Design review of the part built by this model. Coordinates are the model's own, in mm. A direction names the side the tool comes from. Coordinates: 2 decimals unless noted, no trailing zeros. Loops run counter-clockwise (first coordinate to the right, second up) from the corner with the lowest first, then second, coordinate; pieces in that order, holes last. Notation, with made-up numbers: (69, 37) -> (89, 37) arc R14 ccw to (89, 63) -> close; hole circle Ø11 at (-4, 6). An arc over 180 degrees is marked (long way). Use CSV: the item, a comma, the result in double quotes.
```python
from build123d import *

# Parameters (mm, degrees)
BOSS_EXTRUDE1_DEPTH = 10
SKETCH2_R           = 1.85
CUT_EXTRUDE1_DEPTH  = 40
SKETCH2_3_R         = 1.85
CUT_EXTRUDE2_DEPTH  = 40
BOSS_EXTRUDE2_DEPTH = 3


with BuildPart() as part:
    # Sketch1 → Boss-Extrude1 (new body)
    with BuildSketch(Plane.XY):
        Polygon((0, 26), (34.5, 26), (34.5, 0), (45.5, 0), (45.5, 7.020180644), (37.5, 29), (0, 29), align=None)
    extrude(amount=BOSS_EXTRUDE1_DEPTH)

    # Sketch2 → Cut-Extrude1 (cut)
    # profile 1 of 2: a face of its own
    with BuildSketch(Plane(origin=(0, 7.020180644, 0), x_dir=(1, 0, 0), z_dir=(0, 1, 0))):
        Polygon((37, -3.267949192), (37, -6.732050808), (40, -8.464101615), (43, -6.732050808), (43, -3.267949192), (40, -1.535898385), align=None)
        with Locations((40, -5)):
            Circle(SKETCH2_R, mode=Mode.SUBTRACT)
    # profile 2 of 2: a face of its own
    with BuildSketch(Plane(origin=(0, 7.020180644, 0), x_dir=(1, 0, 0), z_dir=(0, 1, 0))):
        with Locations((40, -5)):
            Circle(SKETCH2_R)
    extrude(amount=CUT_EXTRUDE1_DEPTH, mode=Mode.SUBTRACT)

    # Sketch2_3 → Cut-Extrude2 (cut)
    with BuildSketch(Plane(origin=(0, 7.020180644, 0), x_dir=(1, 0, 0), z_dir=(0, 1, 0))):
        with Locations(Location((40, -5, 0), (0, 0, 180))):
            Circle(SKETCH2_3_R)
    extrude(amount=-CUT_EXTRUDE2_DEPTH, mode=Mode.SUBTRACT)

    # Mirror1: part across plane


with BuildPart() as part_1:
    add(part.part)
    add(part.part.mirror(Plane(origin=(0, 29, 10), x_dir=(0, 0, 1), z_dir=(1, 0, 0))))

    # Sketch3 → Boss-Extrude2 (add)
    with BuildSketch(Plane.XY.offset(10)):
        Polygon((31.5, 0), (45.5, 0), (45.5, 7.020180644), (37.5, 29), (-37.5, 29), (-45.5, 7.020180644), (-45.5, 0), (-31.5, 0), (-31.5, 26), (31.5, 26), align=None)
    extrude(amount=BOSS_EXTRUDE2_DEPTH)


solid = part_1.part
```
Item 1: Draft analysis for pull direction X (two halves, no side actions). For faces 1 (the face through (1, 29, 6)), 2 (the face through (-41.15, 12.79, 7.8)), 3 (the face through (-41.85, 3.56, 5.08)), 4 (the face through (45.5, 3, 6)), state which applies: pulls with the +X half, pulls with the -X half, needs draft (parallel to the pull), parting line crosses it, or undercut.
Checked values:
face 1,"needs draft"
face 2,"undercut"
face 3,"undercut"
face 4,"pulls with the +X half"
Item 2: Add section D-D (y = 23.5). Give the boundary of the cut face in (x, z), then the cut area to 3 significant figures.
Checked values:
outline,"(-39.5, 0) -> (-34.5, 0) -> (-34.5, 10) -> (-31.5, 10) -> (-31.5, 13) -> (-39.5, 13) -> (-39.5, 8.18) -> (-37, 6.73) -> (-37, 3.27) -> (-39.5, 1.82) -> close; (31.5, 10) -> (34.5, 10) -> (34.5, 0) -> (39.5, 0) -> (39.5, 1.82) -> (37, 3.27) -> (37, 6.73) -> (39.5, 8.18) -> (39.5, 13) -> (31.5, 13) -> close"
area,"123 mm^2"
Item 3: Clearance check with flat-ended pins moving along their axes: pin 1 (1.8 mm diameter, centred on x = -41.5, z = 5, fed in from +Y); pin 2 (4 mm diameter, centred on y = 11, z = 11.5, fed in from -X); pin 3 (5 mm diameter, centred on y = 13, z = 6, fed in from +X); pin 4 (4 mm diameter, centred on x = 33.5, y = 25, fed in from -Z). State where each tip first meets the part, or that it passes through.
Checked values:
pin 1,"y = 7.02"
pin 2,"x = -44.78"
pin 3,"x = 44.23"
pin 4,"z = 0"
Item 4: Add section A-A (y = 15.5). Give the boundary of the cut face in (x, z), then the cut area to 3 significant figures.
Checked values:
outline,"(-42.41, 0) -> (-34.5, 0) -> (-34.5, 10) -> (-31.5, 10) -> (-31.5, 13) -> (-42.41, 13) -> (-42.41, 7.07) -> (-40, 8.46) -> (-37, 6.73) -> (-37, 3.27) -> (-40, 1.54) -> (-42.41, 2.93) -> close; (31.5, 10) -> (34.5, 10) -> (34.5, 0) -> (42.41, 0) -> (42.41, 2.93) -> (40, 1.54) -> (37, 3.27) -> (37, 6.73) -> (40, 8.46) -> (42.41, 7.07) -> (42.41, 13) -> (31.5, 13) -> close"
area,"166 mm^2"
Item 5: Add section B-B (z = 5). Give the boundary of the cut face in (x, y).
Checked values:
outline,"(-45.5, 0) -> (-41.85, 0) -> (-41.85, 7.02) -> (-43, 7.02) -> (-43, 13.89) -> (-45.5, 7.02) -> close; (-38.15, 0) -> (-34.5, 0) -> (-34.5, 26) -> (34.5, 26) -> (34.5, 0) -> (38.15, 0) -> (38.15, 7.02) -> (37, 7.02) -> (37, 29) -> (-37, 29) -> (-37, 7.02) -> (-38.15, 7.02) -> close; (41.85, 0) -> (45.5, 0) -> (45.5, 7.02) -> (43, 13.89) -> (43, 7.02) -> (41.85, 7.02) -> close"
Item 6: Machinability: for faces 5 (the face through (-45.5, 4, 6)), 6 (the face through (43, 10, 5)), 7 (the face through (-34.5, 13, 5)), 8 (the face through (-40, 0, 8)), 9 (the face through (-31.5, 13, 11)), which of the approach directions +Z, -Z, +X, -X, +Y, -Y give a long, thin tool a straight path to every point of the face, cutting with its end or side? Answer none if there is none.
Checked values:
face 5,"+Z, -Z, -X, +Y, -Y"
face 6,"+Y"
face 7,"-Z, -Y"
face 8,"+Z, -Z, +X, -X, -Y"
face 9,"+Z, -Z, -Y"
Item 7: Add section C-C (y = 11). Give the boundary of the cut face in (x, z), then the cut area to 3 significant figures.
Checked values:
outline,"(-44.05, 0) -> (-34.5, 0) -> (-34.5, 10) -> (-31.5, 10) -> (-31.5, 13) -> (-44.05, 13) -> close; (31.5, 10) -> (34.5, 10) -> (34.5, 0) -> (44.05, 0) -> (44.05, 13) -> (31.5, 13) -> close; hole (-43, 3.27) -> (-40, 1.54) -> (-37, 3.27) -> (-37, 6.73) -> (-40, 8.46) -> (-43, 6.73) -> close; hole (37, 3.27) -> (40, 1.54) -> (43, 3.27) -> (43, 6.73) -> (40, 8.46) -> (37, 6.73) -> close"
area,"204 mm^2"
Item 8: To check wall thickness, follow line 1 along Z through (x, y) = (-40, 5); line 2 along X through (y, z) = (4, 6); line 3 along X through (y, z) = (15, 4.75). State the ranges of each line that lie inside material, in increasing order.
Checked values:
line 1,"0 to 3.15, 6.85 to 13"
line 2,"-45.5 to -41.56, -38.44 to -34.5, 34.5 to 38.44, 41.56 to 45.5"
line 3,"-37 to -34.5, 34.5 to 37"
